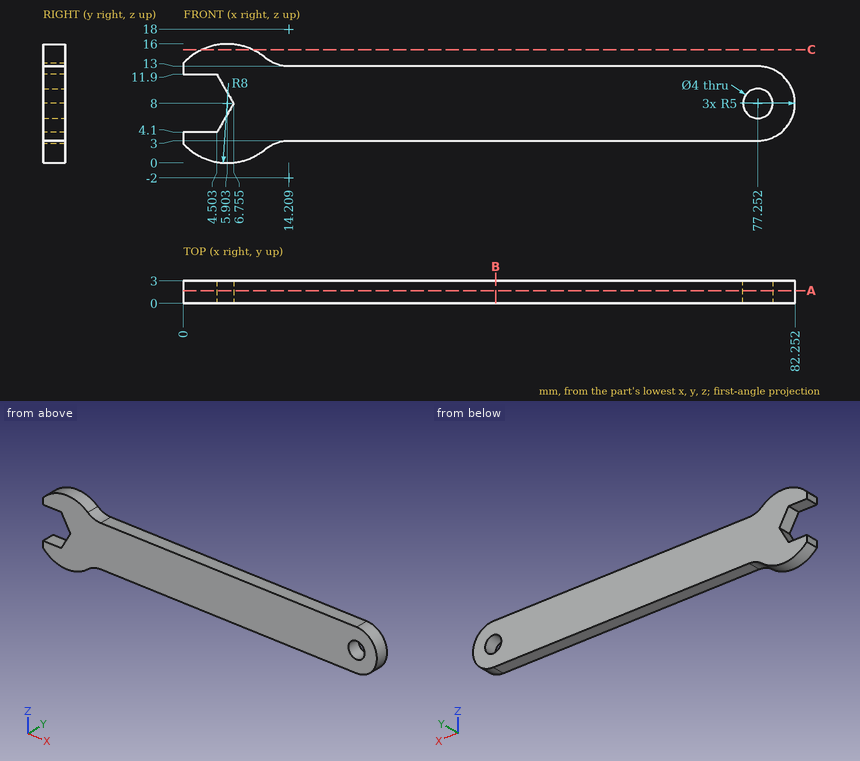
Could you check a few things on this drawing? It's one solid part, dimensions in mm from its lowest x, y, z. Coordinates: 2 decimals unless noted, no trailing zeros. Order: outer loops, then holes, each group sorted by start corner. A loop starts at its lowest first (then second) coordinate and runs counter-clockwise, first axis right, second up.
1. I'm going to push flat-ended pins straight in: pin 1 (1.5 mm diameter, centred on x = 12.5, y = 0.5, fed in from -Z); pin 2 (3.5 mm diameter, centred on x = 77.25, z = 8, fed in from -Y); pin 3 (1 mm diameter, centred on x = 35.5, y = 0.5, fed in from -Z); pin 4 (1.5 mm diameter, centred on x = 2.5, y = 1.5, fed in from +Z). Where does each tip first touch, or does it pass through?
2. I need wall thicknesses on line 1 (Z direction, x = 77, y = 1.75) (1 decimal); line 2 (X direction, y = 2.5, z = 7.75) (1 decimal); line 3 (Z direction, x = 73.5, y = 1). Which ranges of each line are inside material? Lowest first, please.
3. If we section it at B-B (x = 42): Please give me the cut outline in (y, z).
4. If we section it at A-A (y = 1.7): Please give me the cut outline in (x, z) (1 decimal).
5. If we section it at C-C (z = 15.25): Please give me the cut outline in (x, y) (1 decimal).
Entries:
1. pin 1: stops at z = 2.35
1. pin 2: passes through
1. pin 3: stops at z = 3
1. pin 4: stops at z = 15.55
2. line 1: z = 3 to 6, 10 to 13
2. line 2: x = 6.6 to 75.3, 79.2 to 82.2
2. line 3: z = 3 to 13
3. outline: (0, 3) - (3, 3) - (3, 13) - (0, 13) - close
4. outline: (0, 2.6) arc R8 ccw to (11, 1.8) arc R5 cw to (14.2, 3) - (77.3, 3) arc R5 ccw to (77.3, 13) - (14.2, 13) arc R5 cw to (11, 14.2) arc R8 ccw to (0, 13.4) - (0, 11.9) - (4.5, 11.9) - (6.8, 8) - (4.5, 4.1) - (0, 4.1) - close; hole circle Ø4 at (77.3, 8)
5. outline: (2.5, 0) - (9.3, 0) - (9.3, 3) - (2.5, 3) - close
